Geometry: final body of the model. Coordinates: model frame, mm. A direction names the side the tool comes from. Round coordinates to 2 decimals unless told otherwise and drop trailing zeros. Loops run counter-clockwise (first coordinate to the right, second up) from the corner with the lowest first, then second, coordinate; pieces in that order, holes last. Notation, with made-up numbers: (28.5, -22) -> (71.5, -22) arc R22 cw to (71.5, -5) -> close; hole circle Ø1 at (-6, 0.5). An arc over 180 degrees is marked (long way). Answer in a Markdown table with one row per item.
```python
from build123d import *

# Parameters (mm, degrees)
SKETCH1_W           = 13.3
SKETCH1_H           = 13.3
SKETCH1_R           = 1.55
SKETCH1_W_2         = 74.5
BOSS_EXTRUDE1_DEPTH = 6.35
FILLET2_R           = 2
CHAMFER1_SIZE       = 6.5
FILLET3_R           = 5
SKETCH2_W           = 7
SKETCH2_H           = 2
CUT_EXTRUDE1_DEPTH  = 53.609742444
FILLET4_R           = 1


with BuildPart() as part:
    # Sketch1 → Boss-Extrude1 (new body)
    # profile 1 of 2: a face of its own
    with BuildSketch(Plane.XY):
        with Locations((-45.15, 0)):
            Rectangle(SKETCH1_W, SKETCH1_H)
        with Locations((-45.3, 0)):
            Circle(SKETCH1_R, mode=Mode.SUBTRACT)
    # profile 2 of 2: a face of its own
    with BuildSketch(Plane.XY):
        with Locations((-1.25, 0)):
            Rectangle(SKETCH1_W_2, SKETCH1_H)
        with Locations((-8.5, 0)):
            Circle(SKETCH1_R, mode=Mode.SUBTRACT)
    extrude(amount=BOSS_EXTRUDE1_DEPTH)

    # Fillet2
    fillet2_edges = [part.edges().sort_by_distance(p)[0] for p in [
        (36, 6.65, 3.175),
        (-51.8, -6.65, 3.175),
        (-51.8, 6.65, 3.175),
    ]]
    fillet(fillet2_edges, radius=FILLET2_R)

    # Chamfer1
    chamfer1_edges = [part.edges().sort_by_distance(p)[0] for p in [
        (36, -6.65, 3.175),
    ]]
    chamfer(chamfer1_edges, length=CHAMFER1_SIZE)

    # Fillet3
    fillet3_edges = [part.edges().sort_by_distance(p)[0] for p in [
        (36, -0.15, 3.175),
        (29.5, -6.65, 3.175),
    ]]
    fillet(fillet3_edges, radius=FILLET3_R)

    # Sketch2 → Cut-Extrude1 (cut, through all)
    with BuildSketch(Plane.XY.offset(6.35)):
        with Locations((32.5, 5.65)):
            Rectangle(SKETCH2_W, SKETCH2_H)
    extrude(amount=-CUT_EXTRUDE1_DEPTH, mode=Mode.SUBTRACT)

    # Fillet4
    fillet4_edges = [part.edges().sort_by_distance(p)[0] for p in [
        (29, 6.65, 3.175),
        (29, 4.65, 3.175),
        (36, 4.65, 3.175),
    ]]
    fillet(fillet4_edges, radius=FILLET4_R - 0.0001)  # a hair under: the kernel refuses the full size


solid = part.part
```
Item 1: Ray query, L1, parallel to Y at x = -45.3, z = 3; L2, parallel to X at y = 1, z = 4.25. Return the intervals inside material, ascending.
Ans:
| item | result |
|---|---|
| L1 | -6.65 to -1.55, 1.55 to 6.65 |
| L2 | -51.8 to -46.48, -44.12 to -9.68, -7.32 to 35.91 |
Item 2: Section query A-A, the plane x = -45.3. Output: boundary loops of the cut face in (y, z).
Ans:
| item | result |
|---|---|
| outline | (-6.65, 0) -> (-1.55, 0) -> (-1.55, 6.35) -> (-6.65, 6.35) -> close; (1.55, 0) -> (6.65, 0) -> (6.65, 6.35) -> (1.55, 6.35) -> close |
Item 3: Section query C-C, the plane y = 0. Output: boundary loops of the cut face in (x, z), and give its area (3 significant figures).
Ans:
| item | result |
|---|---|
| outline | (-51.8, 0) -> (-46.85, 0) -> (-46.85, 6.35) -> (-51.8, 6.35) -> close; (-43.75, 0) -> (-10.05, 0) -> (-10.05, 6.35) -> (-43.75, 6.35) -> close; (-6.95, 0) -> (35.62, 0) -> (35.62, 6.35) -> (-6.95, 6.35) -> close |
| area | 516 mm2 |
Item 4: Section query B-B, the plane z = 3. State how many separate pieces and enclosed holes the cut face has, and give its area (3 significant figures).
Ans:
| item | result |
|---|---|
| separate pieces | 1 |
| enclosed holes | 2 |
| area | 1,110 mm2 |
Item 5: Mould query, pull axis X, two halves, no side actions, for faces 3 (the cylindrical face through (-46.85, 0.07, 3.13)), 4 (the flat face through (-11, 6.65, 3)), 5 (the cylindrical face through (29.32, -6.28, 3.22)). Classes: released by +X, released by -X, zero draft, split by the parting line, or undercut.
Ans:
| item | result |
|---|---|
| face 3 | undercut |
| face 4 | zero draft |
| face 5 | released by +X |
Item 6: Set-up query: faces 1 (the flat face through (32, 4.65, 3)), 2 (the flat face through (32.77, -3.38, 3.13)). Return all of +Z, -Z, +X, -X, +Y, -Y with unobstructed straight access to the full face (end or side cutting, diameter ignored); none if empty.
Ans:
| item | result |
|---|---|
| face 1 | +Z, -Z, +X, +Y |
| face 2 | +Z, -Z, +X, -Y |
